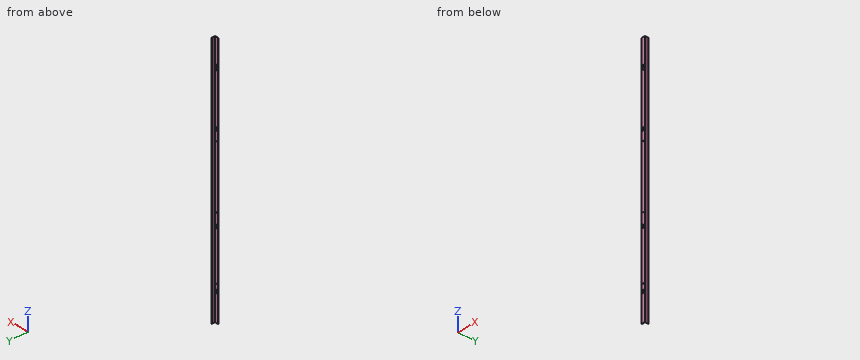
from build123d import *

# Parameters (mm, degrees)
BOSS_EXTRUDE1_DEPTH     = 914.4
F_1_4_20_TAPPED_HOLE1_D = 5.1054
CUT_EXTRUDE1_DEPTH      = 915.798166349


with BuildPart() as part:
    # Sketch2 → Boss-Extrude1 (new, symmetric)
    with BuildSketch(Plane.XY):
        with BuildLine():
            Line((-12.7, -12.7), (12.7, -12.7))
            Line((12.7, -12.7), (12.7, 12.7))
            Line((12.7, 12.7), (11.90625, 12.7))
            ThreePointArc((11.90625, 12.7), (11.344983992, 12.467516008), (11.1125, 11.90625))
            Line((11.1125, 11.90625), (11.1125, -9.5377))
            ThreePointArc((11.1125, -9.5377), (10.651251759, -10.651251759), (9.5377, -11.1125))
            Line((9.5377, -11.1125), (-11.90625, -11.1125))
            ThreePointArc((-11.90625, -11.1125), (-12.467516008, -11.344983992), (-12.7, -11.90625))
            Line((-12.7, -11.90625), (-12.7, -12.7))
        make_face()
    extrude(amount=BOSS_EXTRUDE1_DEPTH, both=True)

    # 1/4-20 Tapped Hole1 (through all)
    with Locations(Plane(origin=(0, -11.1125, 0), x_dir=(1, 0, 0), z_dir=(0, 1, 0))):
        with Locations((-1.5875, -705.104), (-1.5875, -249.428), (-1.5875, 661.924), (-1.5875, 206.248)):
            Hole(F_1_4_20_TAPPED_HOLE1_D / 2)

    # Sketch5 → Cut-Extrude1 (cut, through all)
    with BuildSketch(Plane(origin=(0, -11.1125, 0), x_dir=(1, 0, 0), z_dir=(0, 1, 0))):
        with BuildLine():
            Line((-4.6355, 701.675), (-4.6355, 720.725))
            ThreePointArc((-4.6355, 720.725), (-1.5875, 723.773), (1.4605, 720.725))
            Line((1.4605, 720.725), (1.4605, 701.675))
            ThreePointArc((1.4605, 701.675), (-1.5875, 698.627), (-4.6355, 701.675))
        make_face()
        with BuildLine():
            Line((1.4605, 304.8), (1.4605, 285.75))
            ThreePointArc((1.4605, 285.75), (-1.5875, 282.702), (-4.6355, 285.75))
            Line((-4.6355, 285.75), (-4.6355, 304.8))
            ThreePointArc((-4.6355, 304.8), (-1.5875, 307.848), (1.4605, 304.8))
        make_face()
        with BuildLine():
            Line((1.4605, -336.55), (1.4605, -317.5))
            ThreePointArc((1.4605, -317.5), (-1.5875, -314.452), (-4.6355, -317.5))
            Line((-4.6355, -317.5), (-4.6355, -336.55))
            ThreePointArc((-4.6355, -336.55), (-1.5875, -339.598), (1.4605, -336.55))
        make_face()
        with BuildLine():
            Line((-4.6355, -717.55), (-4.6355, -736.6))
            ThreePointArc((-4.6355, -736.6), (-1.5875, -739.648), (1.4605, -736.6))
            Line((1.4605, -736.6), (1.4605, -717.55))
            ThreePointArc((1.4605, -717.55), (-1.5875, -714.502), (-4.6355, -717.55))
        make_face()
    extrude(amount=-CUT_EXTRUDE1_DEPTH, mode=Mode.SUBTRACT)


solid = part.part
The listing builds one solid part. Answer for the finished solid, in the listing's coordinates (mm). Coordinates: 2 decimals unless noted, no trailing zeros. Write each loop counter-clockwise with the first axis right and the second up, starting at its lowest first coordinate (ties: lowest second). Pieces come first, ordered by that corner, then holes. Notation, with made-up numbers: M 26.25,21 L 42.25,21 A21 cw 42.25,28 Z; hole C 67,-12 d3. An arc over 180 degrees is marked long. Put each result on its own line as item: value. Start each with the question number.
1. Flat-ended cylindrical pins translate along their axes: P1, Ø12, axis at x = -5, z = -429, coming from the +Y side; P2, Ø4.5, axis at x = -1.59, z = -206.25, coming from the +Y side; P3, Ø1, axis at y = -4.5, z = -59.5, coming from the -X side. Find the tip coordinate at first contact, or state that the pin passes through.
2. A cutting plane is placed at A-A on z = -59.5. Write down the section's boundary in (x, y).
3. Consider line 1 (Y direction, x = -1, z = -113.5); line 2 (X direction, y = -6.75, z = -836.5); line 3 (Y direction, x = 11.5, z = 799). Determine where each line is inside the solid, lowest interval first. Write a range as from..to.
4. A cutting plane is placed at B-B on y = 4.5. Write down the section's boundary in (x, z), then the cut area to 3 significant figures.
Resolved:
1. P1: stops at y = -11.11
1. P2: passes through
1. P3: stops at x = 11.11
2. outline: M -12.7,-12.7 L 12.7,-12.7 L 12.7,12.7 L 11.91,12.7 A0.79 ccw 11.11,11.91 L 11.11,-9.54 A1.57 cw 9.54,-11.11 L -11.91,-11.11 A0.79 ccw -12.7,-11.91 Z
3. line 1: y = -12.7..-11.11
3. line 2: x = 11.11..12.7
3. line 3: y = -12.7..12.59
4. outline: M 11.11,-914.4 L 12.7,-914.4 L 12.7,914.4 L 11.11,914.4 Z
4. area: 2,900 mm2
